Here's how the part is built. I have some questions about the finished solid (model axes, mm). A direction names the side the tool comes from. Coordinates: 2 decimals unless noted, no trailing zeros. Loops run counter-clockwise (first coordinate to the right, second up) from the corner with the lowest first, then second, coordinate; pieces in that order, holes last.
from build123d import *

# Parameters (mm, degrees)
PAD_DEPTH       = 45
FILLET_R        = 2
CHAMFER_SIZE    = 5
SKETCH001_R     = 1.8
POCKET_DEPTH    = 5
POCKET001_DEPTH = 5


with BuildPart() as part:
    # Sketch → Pad (new body)
    with BuildSketch(Plane.XY):
        with BuildLine():
            Line((11.154947, 7.919356), (13.654947, 7.919356))
            Line((13.654947, 7.919356), (13.654947, 34.219356))
            Line((13.654947, 34.219356), (-11.345053, 34.219356))
            Line((-11.345053, 34.219356), (-11.345053, -5.780644))
            Line((-11.345053, -5.780644), (-26.345053, -5.780644))
            Line((-26.345053, -5.780644), (-26.345053, -8.280644))
            Line((-26.345053, -8.280644), (-8.845053, -8.280644))
            Line((-8.845053, -8.280644), (-8.845053, 31.719356))
            Line((-8.845053, 31.719356), (11.154947, 31.719356))
            Line((11.154947, 31.719356), (11.154947, 11.919356))
            ThreePointArc((11.154947, 11.919356), (9.154947, 9.919356), (11.154947, 7.919356))
        make_face()
    extrude(amount=PAD_DEPTH)

    # Fillet
    fillet_edges = [part.edges().sort_by_distance(p)[0] for p in [
        (-8.845053, -8.280644, 22.5),
        (-11.345053, -5.780644, 22.5),
        (-11.345053, 34.219356, 22.5),
        (13.654947, 34.219356, 22.5),
        (13.654947, 7.919356, 22.5),
    ]]
    fillet(fillet_edges, radius=FILLET_R)

    # Chamfer
    chamfer_edges = [part.edges().sort_by_distance(p)[0] for p in [
        (-26.345053, -7.030644, 0),
        (-26.345053, -7.030644, 45),
    ]]
    chamfer(chamfer_edges, length=CHAMFER_SIZE)

    # Sketch001 (on Face2 of Chamfer) → Pocket (cut)
    with BuildSketch(Plane.XZ.offset(8.280644)):
        with Locations((-20.345053, 4.25)):
            Circle(SKETCH001_R)
        with Locations((-20.345053, 40.75)):
            Circle(SKETCH001_R)
    extrude(amount=-POCKET_DEPTH, mode=Mode.SUBTRACT)

    # Sketch002 (on Face2 of Pocket) → Pocket001 (cut)
    with BuildSketch(Plane.XZ.offset(8.280644)):
        with BuildLine():
            ThreePointArc((-23.702854, 1.362278), (-15.565, 8.554641), (-21.702854, 17.514636))
            Line((-21.702854, 17.514636), (-26.750495, 22.562278))
            Line((-26.750495, 22.562278), (-21.702854, 27.60992))
            ThreePointArc((-21.702854, 27.60992), (-15.565, 36.569915), (-23.702854, 43.762278))
            Line((-23.702854, 43.762278), (-32.41938, 43.762278))
            Line((-32.41938, 43.762278), (-32.41938, 1.362278))
            Line((-32.41938, 1.362278), (-23.702854, 1.362278))
        make_face()
        with BuildLine():
            ThreePointArc((-14.302854, 26.062278), (-16.202854, 27.962278), (-18.102854, 26.062278))
            Line((-18.102854, 26.062278), (-18.102854, 19.062278))
            ThreePointArc((-18.102854, 19.062278), (-16.202854, 17.162278), (-14.302854, 19.062278))
            Line((-14.302854, 26.062278), (-14.302854, 19.062278))
        make_face()
    extrude(amount=-POCKET001_DEPTH, mode=Mode.SUBTRACT)


solid = part.part
Q1. For faces 1 (the cylindrical face through (9.155, 9.963, 22.185)), 2 (the flat face through (-18.3, -5.781, 22.2)), 3 (the cylindrical face through (-16.245, -7.048, 17.163)), which set-ups out of +Z, -Z, +X, -X, +Y, -Y let a thin tool reach every point of the face, with its end or its side?
Q2. We'd pull the mould along X, two halves only. Please class faces 4 (the cylindrical face through (13.1, 33.6, 22.8)), 5 (the flat face through (11.155, 22, 22)), 6 (the flat face through (-22.007, -7.013, 44.338)): pulls with the +X half, pulls with the -X half, needs draft (parallel to the pull), parting line crosses it, or undercut.
Q3. Suppose I cut it at D-D on z = 24.5. Write out the boundary of the cut face in (x, y), and give its area (3 significant figures).
Q4. Please list where these lines run through material, in increasing order: probe 1 along X at (y, z) = (27, 33); probe 2 along Y at (x, z) = (-3.5, 17.5); probe 3 along X at (y, z) = (6.5, 21.5).
Q5. Suppose I cut it at A-A on y = 24.5. Write out the boundary of the cut face in (x, z).
Q6. Will these pins go through, and if not, where does the flat tip stop? P1, Ø14.5, axis at x = -21, z = 16, coming from the +Y side; P2, Ø0.8, axis at y = -7, z = 23, coming from the +X side; P3, Ø3, axis at y = 0, z = 18.5, coming from the +X side.
Q7. Suppose I cut it at B-B on x = -20.5. Write out the boundary of the cut face in (y, z), and give its area (3 significant figures).
Q8. Suppose I cut it at C-C on x = 10. Write out the boundary of the cut face in (y, z).
Check values:
1. face 1: +Z, -Z
1. face 2: +Z, -Z, -X, +Y
1. face 3: +Y, -Y
2. face 4: pulls with the +X half
2. face 5: undercut
2. face 6: pulls with the -X half
3. outline: (-24.81, -8.28) - (-18.1, -8.28) - (-18.1, -5.78) - (-24.81, -5.78) - close; (-14.3, -8.28) - (-10.85, -8.28) arc R2 ccw to (-8.85, -6.28) - (-8.85, 31.72) - (11.15, 31.72) - (11.15, 11.92) arc R2 ccw to (11.15, 7.92) - (11.65, 7.92) arc R2 ccw to (13.65, 9.92) - (13.65, 32.22) arc R2 ccw to (11.65, 34.22) - (-9.35, 34.22) arc R2 ccw to (-11.35, 32.22) - (-11.35, -3.78) arc R2 cw to (-13.35, -5.78) - (-14.3, -5.78) - close
3. area: 250 mm2
4. probe 1: x = -11.35 to -8.85, 11.15 to 13.65
4. probe 2: y = 31.72 to 34.22
4. probe 3: x = -11.35 to -8.85
5. outline: (-11.35, 0) - (-8.85, 0) - (-8.85, 45) - (-11.35, 45) - close; (11.15, 0) - (13.65, 0) - (13.65, 45) - (11.15, 45) - close
6. P1: stops at y = -5.78
6. P2: stops at x = -8.87
6. P3: stops at x = -8.85
7. outline: (-8.28, 0) - (-5.78, 0) - (-5.78, 2.01) - (-8.28, 2.01) - close; (-8.28, 17.11) - (-5.78, 17.11) - (-5.78, 28.01) - (-8.28, 28.01) - close; (-8.28, 43.11) - (-5.78, 43.11) - (-5.78, 45) - (-8.28, 45) - close
7. area: 37.0 mm2
8. outline: (8.29, 0) - (11.55, 0) - (11.55, 45) - (8.29, 45) - close; (31.72, 0) - (34.22, 0) - (34.22, 45) - (31.72, 45) - close
